Geometry check sheet. Reference: the model listing, model coordinates, mm. A direction names the side the tool comes from. Round coordinates to 2 decimals unless told otherwise and drop trailing zeros. Write each loop counter-clockwise with the first axis right and the second up, starting at its lowest first coordinate (ties: lowest second). Pieces come first, ordered by that corner, then holes. Notation, with made-up numbers: (35, 21.5) -> (62, 21.5) arc R22 ccw to (62, 42.5) -> close; hole circle Ø4 at (38.5, 67). An arc over 180 degrees is marked (long way). Use a Markdown table: item, result.
Autodesk Inventor part; units mm, degrees
ref_plane "YZ Plane" through (0, 0, 0) normal (1, 0, 0) x (0, 1, 0)
ref_plane "XZ Plane" through (0, 0, 0) normal (0, 1, 0) x (-1, 0, 0)
ref_plane "XY Plane" through (0, 0, 0) normal (0, 0, 1) x (1, 0, 0)
sketch "Szkic1" plane through (0, 0, 0) normal (0, 1, 0) x (-1, 0, 0)
  line L0 (0, 0) -> (0, -53.4)
  line L1 (0, -53.4) -> (113, -53.4)
  line L2 (0, -53.4) -> (113, -53.4) construction
  line L3 (0, -53.4) -> (113, -53.4)
  line L4 (113, -53.4) -> (113, 0)
  line L5 (113, 0) -> (0, 0)
  line L6 (0, 0) -> (0, -53.4)
  dimension "d0" = 53.4
  dimension "d1" = 113
  dimension "d2" = 0
extrude "Wyciągnięcie proste1" add sketch "Szkic1" along normal blind 1
sketch "Szkic2" plane through (0, 1, 0) normal (0, 1, 0) x (1, 0, 0)
  line L0 (-113, 53.4) -> (-113, 0)
  line L1 (-113, 0) -> (-83, 0)
  line L2 (-113, 0) -> (0, 0)
  line L3 (-83, 0) -> (-83, 53.4)
  line L4 (0, 53.4) -> (-113, 53.4)
  line L5 (-83, 0) -> (0, 0)
  line L6 (0, 0) -> (0, 53.4)
  line L7 (0, 53.4) -> (-83, 53.4)
  line L8 (-83, 53.4) -> (-83, 0)
  line L9 (-83, 0) -> (-79, 0)
  line L10 (-79, 0) -> (-79, 4)
  line L11 (0, 53.4) -> (-4, 53.4)
  line L12 (-4, 53.4) -> (-4, 49.4)
  line L13 (-79, 4) -> (-4, 4)
  line L14 (-4, 4) -> (-4, 49.4)
  line L15 (-4, 49.4) -> (-79, 49.4)
  line L16 (-79, 49.4) -> (-79, 4)
  dimension "d5" = 30
  dimension "d6" = 4
  dimension "d7" = 4
  dimension "d8" = 4
  dimension "d9" = 4
extrude "Wyciągnięcie proste2" add sketch "Szkic2" along normal blind 13 contours L4 L12 L15 L16 L10 L2 L3 | L4 L6 L2 L10 L13 L14 L12
sketch "Szkic3" plane through (0, 1, 0) normal (0, 1, 0) x (1, 0, 0)
  line L0 (-113, 53.4) -> (-113, 0)
  line L1 (-113, 26.7) -> (-113, 12.05)
  line L2 (-113, 26.7) -> (-113, 41.35)
  arc A0 (-113, 12.05) -> (-113, 41.35) centre (-115.5542, 26.7) ccw
  point P0 (0, 0)
  dimension "d12" = 14.65
  dimension "d13" = 14.65
  dimension "d14" = 14.871
extrude "Wyciągnięcie proste3" cut sketch "Szkic3" against normal blind 13
chamfer "Faza1" distance 13 angle 45 1 edges at (-83, 1, -26.7)
sketch "Szkic4" plane through (-79, 1, -4) normal (1, 0, 0) x (0, 0, -1)
  line L0 (45.4, 0) -> (0, 0)
  line L1 (22.7, 0) -> (22.7, 13)
  line L2 (0, 13) -> (45.4, 13)
  circle A0 centre (22.7, 6.5) radius 6
  point P0 (-4, -1)
  dimension "d20" = 12
extrude "Wyciągnięcie proste4" cut sketch "Szkic4" against normal through all
sketch "Szkic5" plane through (0, 0, 0) normal (1, 0, 0) x (0, 0, -1)
  line L0 (0, 0) -> (0, 14)
  line L1 (0, 7) -> (53.4, 7)
  line L2 (53.4, 0) -> (53.4, 14)
  line L3 (4, 14) -> (49.4, 14)
  line L4 (26.7, 14) -> (26.7, 0)
  line L5 (0, 0) -> (53.4, 0)
  circle A0 centre (26.7, 7) radius 2
  line L6 (26.7, 9) -> (26.7, 10)
  line L7 (26.7, 10) -> (26.7, 12) construction
  line L8 (27.45, 10) -> (27.45, 12)
  line L9 (25.95, 12) -> (25.95, 10)
  arc A1 (25.95, 10) -> (27.45, 10) centre (26.7, 10) ccw
  arc A2 (27.45, 12) -> (25.95, 12) centre (26.7, 12) ccw
  line L10 (28.1142, 8.4142) -> (28.8213, 9.1213)
  line L11 (28.8213, 9.1213) -> (30.2355, 10.5355) construction
  line L12 (29.7052, 11.0659) -> (28.291, 9.6517)
  arc A3 (28.291, 9.6517) -> (29.3517, 8.591) centre (28.8213, 9.1213) ccw
  arc A4 (30.7659, 10.0052) -> (29.7052, 11.0659) centre (30.2355, 10.5355) ccw
  line L13 (29.3517, 8.591) -> (30.7659, 10.0052)
  line L14 (28.7, 7) -> (29.7, 7)
  line L15 (29.7, 7) -> (31.7, 7) construction
  line L16 (31.7, 7.75) -> (29.7, 7.75)
  arc A5 (29.7, 7.75) -> (29.7, 6.25) centre (29.7, 7) ccw
  arc A6 (31.7, 6.25) -> (31.7, 7.75) centre (31.7, 7) ccw
  line L17 (29.7, 6.25) -> (31.7, 6.25)
  line L18 (28.1142, 5.5858) -> (28.8213, 4.8787)
  line L19 (28.8213, 4.8787) -> (30.2355, 3.4645) construction
  line L20 (30.7659, 3.9948) -> (29.3517, 5.409)
  arc A7 (29.3517, 5.409) -> (28.291, 4.3483) centre (28.8213, 4.8787) ccw
  arc A8 (29.7052, 2.9341) -> (30.7659, 3.9948) centre (30.2355, 3.4645) ccw
  line L21 (28.291, 4.3483) -> (29.7052, 2.9341)
  line L22 (26.7, 5) -> (26.7, 4)
  line L23 (26.7, 4) -> (26.7, 2) construction
  line L24 (27.45, 2) -> (27.45, 4)
  arc A9 (27.45, 4) -> (25.95, 4) centre (26.7, 4) ccw
  arc A10 (25.95, 2) -> (27.45, 2) centre (26.7, 2) ccw
  line L25 (25.95, 4) -> (25.95, 2)
  line L26 (25.2858, 5.5858) -> (24.5787, 4.8787)
  line L27 (24.5787, 4.8787) -> (23.1645, 3.4645) construction
  line L28 (23.6948, 2.9341) -> (25.109, 4.3483)
  arc A11 (25.109, 4.3483) -> (24.0483, 5.409) centre (24.5787, 4.8787) ccw
  arc A12 (22.6341, 3.9948) -> (23.6948, 2.9341) centre (23.1645, 3.4645) ccw
  line L29 (24.0483, 5.409) -> (22.6341, 3.9948)
  line L30 (24.7, 7) -> (23.7, 7)
  line L31 (23.7, 7) -> (21.7, 7) construction
  line L32 (21.7, 6.25) -> (23.7, 6.25)
  arc A13 (23.7, 6.25) -> (23.7, 7.75) centre (23.7, 7) ccw
  arc A14 (21.7, 7.75) -> (21.7, 6.25) centre (21.7, 7) ccw
  line L33 (23.7, 7.75) -> (21.7, 7.75)
  line L34 (25.2858, 8.4142) -> (24.5787, 9.1213)
  line L35 (24.5787, 9.1213) -> (23.1645, 10.5355) construction
  line L36 (22.6341, 10.0052) -> (24.0483, 8.591)
  arc A15 (24.0483, 8.591) -> (25.109, 9.6517) centre (24.5787, 9.1213) ccw
  arc A16 (23.6948, 11.0659) -> (22.6341, 10.0052) centre (23.1645, 10.5355) ccw
  line L37 (25.109, 9.6517) -> (23.6948, 11.0659)
  point P0 (26.7, 11)
  point P1 (29.5284, 9.8284)
  point P2 (30.7, 7)
  point P3 (29.5284, 4.1716)
  point P4 (26.7, 3)
  point P5 (23.8716, 4.1716)
  point P6 (22.7, 7)
  point P7 (23.8716, 9.8284)
  dimension "d23" = 4
  dimension "d24" = 1
  dimension "d25" = 2
  dimension "d26" = 1.5
  dimension "d29" = 360
extrude "Wyciągnięcie proste5" cut sketch "Szkic5" against normal blind 10 contours A15 L36 A16 L37 | A1 L9 A2 L4 | L4 A2 L8 A1 | A3 L12 A4 L13 | A11 L28 A12 L29 | A7 L20 A8 L21 | A14 L33 A13 L1 | L1 A13 L32 A14 | A10 L25 A9 L4 | L4 A9 L24 A10 | A6 L17 A5 L1 | L1 A5 L16 A6
sketch "Szkic6" plane through (0, 1, 0) normal (0, 1, 0) x (1, 0, 0)
  line L0 (-4, 4) -> (-4, 49.4)
  line L1 (-4, 4) -> (-4, 9)
  line L2 (-4, 9) -> (-9, 9)
  line L3 (-9, 9) -> (-19, 9) construction
  line L4 (-9, 11.5) -> (-19, 11.5)
  line L5 (-19, 6.5) -> (-9, 6.5)
  arc A0 (-9, 6.5) -> (-9, 11.5) centre (-9, 9) ccw
  arc A1 (-19, 11.5) -> (-19, 6.5) centre (-19, 9) ccw
  line L6 (-4, 26.7) -> (-79, 26.7)
  line L7 (-79, 49.4) -> (-79, 4)
  line L8 (-79, 4) -> (-4, 4)
  line L9 (-41.5, 4) -> (-41.5, 49.4)
  line L10 (-4, 49.4) -> (-79, 49.4)
  line L11 (-74, 9) -> (-64, 9) construction
  line L12 (-74, 11.5) -> (-64, 11.5)
  line L13 (-64, 6.5) -> (-74, 6.5)
  arc A2 (-74, 11.5) -> (-74, 6.5) centre (-74, 9) ccw
  arc A3 (-64, 6.5) -> (-64, 11.5) centre (-64, 9) ccw
  line L14 (-4, 44.4) -> (-9, 44.4)
  line L15 (-9, 44.4) -> (-19, 44.4) construction
  line L16 (-9, 41.9) -> (-19, 41.9)
  line L17 (-19, 46.9) -> (-9, 46.9)
  arc A4 (-9, 41.9) -> (-9, 46.9) centre (-9, 44.4) ccw
  arc A5 (-19, 46.9) -> (-19, 41.9) centre (-19, 44.4) ccw
  line L18 (-41.5, 49.4) -> (-41.5, 4)
  arc A6 (-74, 46.9) -> (-74, 41.9) centre (-74, 44.4) ccw
  line L19 (-74, 44.4) -> (-64, 44.4) construction
  line L20 (-64, 46.9) -> (-74, 46.9)
  line L21 (-74, 41.9) -> (-64, 41.9)
  arc A7 (-64, 41.9) -> (-64, 46.9) centre (-64, 44.4) ccw
  point P0 (0, 0)
  point P1 (-14, 9)
  point P2 (-69, 9)
  point P3 (-14, 44.4)
  point P4 (-69, 44.4)
  dimension "d33" = 5
  dimension "d34" = 5
  dimension "d35" = 10
  dimension "d36" = 5
extrude "Wyciągnięcie proste6" cut sketch "Szkic6" against normal blind 10 contours A0 L5 A1 L4 | A4 L16 A5 L17 | L12 A3 L13 A2 | L20 A7 L21 A6
sketch "Szkic7" plane through (0, 0, -53.4) normal (0, 0, -1) x (-1, 0, 0)
  line L0 (79, 1) -> (4, 1)
  line L1 (41.5, 1) -> (41.5, 14)
  line L2 (4, 14) -> (79, 14)
  line L3 (79, 1.5) -> (79, 13.5)
  line L4 (79, 7.5) -> (41.5, 7.5)
  line L5 (41.5, 7.5) -> (31.5, 7.5)
  line L6 (31.5, 7.5) -> (51.5, 7.5) construction
  line L7 (31.5, 3) -> (51.5, 3)
  line L8 (51.5, 12) -> (31.5, 12)
  arc A0 (31.5, 12) -> (31.5, 3) centre (31.5, 7.5) ccw
  arc A1 (51.5, 3) -> (51.5, 12) centre (51.5, 7.5) ccw
  point P0 (0, 0)
  dimension "d39" = 10
  dimension "d40" = 20
  dimension "d41" = 9
extrude "Wyciągnięcie proste7" cut sketch "Szkic7" against normal blind 10
properties part number "klp"
(1) Thickness scan on line 1 (Z direction, x = -88.5, y = 7.5); line 2 (Z direction, x = -19, y = 1.75); line 3 (Y direction, x = -80, z = -27). Record the ranges inside material, lowest first.
A:
| item | result |
|---|---|
| line 1 | z = -53.4 to -32.7, -20.7 to 0 |
| line 2 | z = -53.4 to -49.4, -4 to 0 |
| line 3 | y = 0 to 1.51, 13.49 to 14 |
(2) Gauge pin test, flat ends, axial feed: pin 1 Ø22.5 at (x, z) = (-46, -25.5) entering from +Y; pin 2 Ø3 at (y, z) = (12.5, -34.5) entering from -X. Record the tip position at first contact, or that the pin passes through.
A:
| item | result |
|---|---|
| pin 1 | stops at y = 1 |
| pin 2 | stops at x = -86 |
(3) Access from +Z, -Z, +X, -X, +Y, -Y to the whole of each face (thin tool, end or side, straight path). Record for faces 4 (the face through (-6.5, 0.5, -44.3)), 5 (the face through (-2, 7.75, -23)), 6 (the face through (-41, 1, -26)).
A:
| item | result |
|---|---|
| face 4 | +Y, -Y |
| face 5 | +X, -X |
| face 6 | +Y |
(4) Release check for a two-part mould opening along Z. For faces 1 (the face through (-2, 3, -25.95)), 2 (the face through (-27, 7.6, -51.4)), 3 (the face through (-45, 7, 0)) record: +Z half, -Z half, draft (parallel to the pull), parting line (faces both ways), or undercut.
A:
| item | result |
|---|---|
| face 1 | undercut |
| face 2 | draft |
| face 3 | +Z half |
(5) Section check A-A on x = -16.5. Record the cut outline in (y, z).
A:
| item | result |
|---|---|
| outline | (0, -53.4) -> (14, -53.4) -> (14, -49.4) -> (1, -49.4) -> (1, -46.9) -> (0, -46.9) -> close; (0, -41.9) -> (1, -41.9) -> (1, -11.5) -> (0, -11.5) -> close; (0, -6.5) -> (1, -6.5) -> (1, -4) -> (14, -4) -> (14, 0) -> (0, 0) -> close |
(6) Section check C-C on x = -97.5. Record the cut outline in (y, z), plus the area to 3 significant figures.
A:
| item | result |
|---|---|
| outline | (0, -53.4) -> (1, -53.4) -> (1, 0) -> (0, 0) -> close |
| area | 53.4 mm2 |
